```python
from build123d import *

# Parameters (mm, degrees)
PAD_DEPTH               = 21
PAD001_DEPTH            = 5
PAD_MIRRORED_2_DEPTH    = 21
PAD001_MIRRORED_2_DEPTH = 5


with BuildPart() as part:
    # Sketch → Pad (new body)
    with BuildSketch(Plane.XY):
        with BuildLine():
            ThreePointArc((9, 0), (6.363961, 6.363961), (0, 9))
            Line((0, 9), (0, 24.941391))
            Line((0, 24.941391), (31.444139, 24.941391))
            Line((31.444139, 24.941391), (31.444139, 0))
            Line((31.444139, 0), (9, 0))
        make_face()
    pad = extrude(amount=PAD_DEPTH)

    # Sketch001 → Pad001 (join)
    with BuildSketch(Plane.XY):
        with BuildLine():
            ThreePointArc((9, 0), (6.363961, 6.363961), (0, 9))
            Line((0, 9), (0, 4))
            ThreePointArc((4, 0), (2.828427, 2.828427), (0, 4))
            Line((4, 0), (9, 0))
        make_face()
    pad001 = extrude(amount=PAD001_DEPTH)

    # Sketch Mirrored 2 → Pad Mirrored 2 (add)
    with BuildSketch(Plane(origin=(0, 0, 0), x_dir=(-1, 0, 0), z_dir=(0, 0, -1))):
        with BuildLine():
            ThreePointArc((9, 0), (6.363961, 6.363961), (0, 9))
            Line((0, 9), (0, 24.941391))
            Line((0, 24.941391), (31.444139, 24.941391))
            Line((31.444139, 24.941391), (31.444139, 0))
            Line((31.444139, 0), (9, 0))
        make_face()
    pad_mirrored_2 = extrude(amount=-PAD_MIRRORED_2_DEPTH)

    # Sketch001 Mirrored 2 → Pad001 Mirrored 2 (add)
    with BuildSketch(Plane(origin=(0, 0, 0), x_dir=(-1, 0, 0), z_dir=(0, 0, -1))):
        with BuildLine():
            ThreePointArc((9, 0), (6.363961, 6.363961), (0, 9))
            Line((0, 9), (0, 4))
            ThreePointArc((4, 0), (2.828427, 2.828427), (0, 4))
            Line((4, 0), (9, 0))
        make_face()
    pad001_mirrored_2 = extrude(amount=-PAD001_MIRRORED_2_DEPTH)

    # Mirrored001: Pad, Pad001, Pad Mirrored 2, Pad001 Mirrored 2 across Sketch H_Axis
    add(pad.mirror(Plane.ZX))
    add(pad001.mirror(Plane.ZX))
    add(pad_mirrored_2.mirror(Plane.ZX))
    add(pad001_mirrored_2.mirror(Plane.ZX))


with BuildPart() as part_1:
    # Clone placement: moved
    add(part.part.moved(Location((395, 362, -21))))


solid = part_1.part
```
Could you check a few things on this model? Use its own coordinates, in mm. Give positions to 0.01 mm unless a question says otherwise; leave off trailing zeros. Loops run counter-clockwise (first coordinate to the right, second up) from the corner with the lowest first, then second, coordinate; pieces in that order, holes last. Notation, with made-up numbers: (45, -11.75) - (83, -11.75) arc R7 cw to (83, 1.25) - close; hole circle Ø5 at (59.25, 64). An arc over 180 degrees is marked (long way). Answer in a Markdown table with one row per item. Add a question column.
Q1. For pin 1 (5.5 mm diameter, centred on x = 399, y = 359, fed in from +Z), with a flat end and sliding along its axis, tell me the tip position at first contact or that it passes through.
Q2. If we section it at C-C (x = 388): List the corners of the cut face in (y, z) for me, plus the area to 3 significant figures.
Q3. If we section it at D-D (z = -17): List the corners of the cut face in (x, y) for me, plus the area to 3 significant figures.
Q4. Please list where these lines run through material, in increasing order: L1, parallel to X at y = 362.5, z = -6.75; L2, parallel to X at y = 369.5, z = -3.25; L3, parallel to Y at x = 402, z = -15.5. Write a range as from..to.
Q5. We'd pull the mould along Y, two halves only. Please class faces 1 (the face through (395, 356, -21)), 2 (the face through (395, 386.941, -11)), 3 (the face through (393, 366, -16)): +Y half, -Y half, draft (parallel to the pull), parting line (faces both ways), or undercut.
Q6. If we section it at B-B (y = 367): List the corners of the cut face in (x, z) for me.
Q7. If we section it at A-A (z = -7): List the corners of the cut face in (x, y) for me.
The answers:
| question | item | result |
|---|---|---|
| 1 | pin 1 | stops at z = -16 |
| 2 | outline | (337.06, -21) - (386.94, -21) - (386.94, 0) - (367.66, 0) - (367.66, -16) - (356.34, -16) - (356.34, 0) - (337.06, 0) - close |
| 2 | area | 867 mm^2 |
| 3 | outline | (363.56, 337.06) - (426.44, 337.06) - (426.44, 386.94) - (363.56, 386.94) - close; hole circle Ø8 at (395, 362) |
| 3 | area | 3,090 mm^2 |
| 4 | L1 | x = 363.56..386.01, 403.99..426.44 |
| 4 | L2 | x = 363.56..390.03, 399.97..426.44 |
| 4 | L3 | y = 337.06..356.34, 367.66..386.94 |
| 5 | face 1 | draft |
| 5 | face 2 | +Y half |
| 5 | face 3 | undercut |
| 6 | outline | (363.56, -21) - (426.44, -21) - (426.44, 0) - (402.48, 0) - (402.48, -16) - (387.52, -16) - (387.52, 0) - (363.56, 0) - close |
| 7 | outline | (363.56, 337.06) - (426.44, 337.06) - (426.44, 386.94) - (363.56, 386.94) - close; hole circle Ø18 at (395, 362) |
